```python
from build123d import *

# Parameters (mm, degrees)
SKETCH_1_R               = 0.85
EXTRUDE_1_DEPTH          = 1.5
SKETCH_3_R               = 1.175
CUT_EXTRUDE_2_DEPTH      = 1
CUT_EXTRUDE_2_DEPTH_BACK = 4
CHAMFER_1_SIZE           = 0.6


with BuildPart() as part:
    # 草图1 → 凸台-拉伸1 (new body, symmetric)
    with BuildSketch(Plane(origin=(0, 0, 0), x_dir=(0, 0, -1), z_dir=(1, 0, 0))):
        with BuildLine():
            Line((-18, 3.5), (18, 3.5))
            ThreePointArc((18, 3.5), (21.5, 0), (18, -3.5))
            Line((18, -3.5), (-18, -3.5))
            ThreePointArc((-18, -3.5), (-21.5, 0), (-18, 3.5))
        make_face()
        with Locations((18, 0)):
            Circle(SKETCH_1_R, mode=Mode.SUBTRACT)
        with Locations((4, 0)):
            Circle(SKETCH_1_R, mode=Mode.SUBTRACT)
        with Locations((-18, 0)):
            Circle(SKETCH_1_R, mode=Mode.SUBTRACT)
    extrude(amount=EXTRUDE_1_DEPTH, both=True)

    # 草图3 → 切除-拉伸2 (cut, two sides)
    with BuildSketch(Plane.ZY.offset(1.5)) as cut_extrude_2_sk:
        with Locations((-18, 0)):
            Circle(SKETCH_3_R)
        with Locations((-4, 0)):
            Circle(SKETCH_3_R)
        with Locations((18, 0)):
            Circle(SKETCH_3_R)
    extrude(amount=CUT_EXTRUDE_2_DEPTH, mode=Mode.SUBTRACT)
    extrude(cut_extrude_2_sk.sketch, amount=-CUT_EXTRUDE_2_DEPTH_BACK, mode=Mode.SUBTRACT)

    # 倒角1
    chamfer_1_edges = [part.edges().sort_by_distance(p)[0] for p in [
        (1.5, 0, -21.5),
        (1.5, 3.5, 0),
        (1.5, 0, 21.5),
        (-1.5, 3.5, 0),
        (-1.5, 0, -21.5),
        (-1.5, -3.5, 0),
        (-1.5, 0, 21.5),
        (1.5, -3.5, 0),
    ]]
    chamfer(chamfer_1_edges, length=CHAMFER_1_SIZE)


solid = part.part
```
Geometry check sheet. Reference: the model listing, model coordinates, mm. Give positions to 0.01 mm unless a question says otherwise; leave off trailing zeros. Order: outer loops, then holes, each group sorted by start corner. A loop starts at its lowest first (then second) coordinate and runs counter-clockwise, first axis right, second up. Notation, with made-up numbers: (4.5, 49) - (51.5, 49) arc R15 cw to (51.5, 56) - close; hole circle Ø2 at (30.25, -18.5). An arc over 180 degrees is marked (long way). Answer in a Markdown table with one row per item. Add a question column.
Q1. Cross-section at A-A, the plane y = 0. Enter the section's corners in (x, z) (3 decimals).
Q2. Gauge pin test, flat end, axial feed: pin 1 (1.5 mm diameter, centred on x = 1, y = -1, fed in from +Z). Record the tip position at first contact, or that the pin passes through.
Q3. Cross-section at B-B, the plane z = -4. Enter the section's corners in (x, y) (3 decimals).
Q4. Cross-section at C-C, the plane z = 10. Enter the section's corners in (x, y).
Q5. Mould release check, pull along Y, two halves, no side actions. Record for faces 1 (the cylindrical face through (-0.02, 0.35, 19.12)), 2 (the cylindrical face through (-0.02, 0.35, -16.88)), 3 (the conical face through (1.3, 0.1, -21.1)), 4 (the flat face through (0, -3.5, 0)): pulls with the +Y half, pulls with the -Y half, needs draft (parallel to the pull), parting line crosses it, or undercut.
Q6. Material ranges on probe 1 along Y at (x, z) = (0.4, 18) (3 decimals); probe 2 along Z at (x, y) = (0.95, -0.5); probe 3 along Z at (x, y) = (-0.1, -0.5), recorded low to high. Write a range as from..to.
Check values:
| question | item | result |
|---|---|---|
| 1 | outline | (-1.5, -20.9) - (-0.9, -21.5) - (0.9, -21.5) - (1.5, -20.9) - (1.5, -19.175) - (-1.5, -19.175) - close; (-1.5, -16.825) - (1.5, -16.825) - (1.5, -5.175) - (-1.5, -5.175) - close; (-1.5, -2.825) - (1.5, -2.825) - (1.5, 16.825) - (-1.5, 16.825) - close; (-1.5, 19.175) - (1.5, 19.175) - (1.5, 20.9) - (0.9, 21.5) - (-0.9, 21.5) - (-1.5, 20.9) - close |
| 2 | pin 1 | stops at z = 21.49 |
| 3 | outline | (-1.5, -2.9) - (-0.9, -3.5) - (0.9, -3.5) - (1.5, -2.9) - (1.5, -1.175) - (-1.5, -1.175) - close; (-1.5, 1.175) - (1.5, 1.175) - (1.5, 2.9) - (0.9, 3.5) - (-0.9, 3.5) - (-1.5, 2.9) - close |
| 4 | outline | (-1.5, -2.9) - (-0.9, -3.5) - (0.9, -3.5) - (1.5, -2.9) - (1.5, 2.9) - (0.9, 3.5) - (-0.9, 3.5) - (-1.5, 2.9) - close |
| 5 | face 1 | undercut |
| 5 | face 2 | undercut |
| 5 | face 3 | parting line crosses it |
| 5 | face 4 | pulls with the -Y half |
| 6 | probe 1 | y = -3.5..-1.175, 1.175..3.5 |
| 6 | probe 2 | z = -21.41..-19.06, -16.94..-5.06, -2.94..16.94, 19.06..21.41 |
| 6 | probe 3 | z = -21.46..-19.06, -16.94..-5.06, -2.94..16.94, 19.06..21.46 |
